Here's how the part is built. I have some questions about the finished solid (model axes, mm). Face numbers are marked on the shaded views. A direction names the side the tool comes from. Coordinates: 2 decimals unless noted, no trailing zeros. Order: outer loops, then holes, each group sorted by start corner. A loop starts at its lowest first (then second) coordinate and runs counter-clockwise, first axis right, second up.
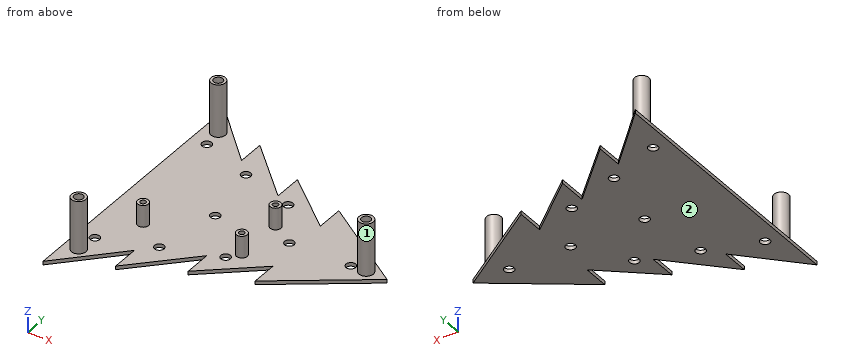
```python
from build123d import *

# Parameters (mm, degrees)
CYLINDER020_R     = 2.55
CYLINDER020_DEPTH = 12
CYLINDER010_R     = 4
CYLINDER010_DEPTH = 31
CYLINDER019_R     = 2.55
CYLINDER019_DEPTH = 12
CYLINDER009_R     = 4
CYLINDER009_DEPTH = 31
CYLINDER018_R     = 2.55
CYLINDER018_DEPTH = 12
CYLINDER011_R     = 4
CYLINDER011_DEPTH = 31
CYLINDER015_R     = 1.55
CYLINDER015_DEPTH = 13
CYLINDER012_R     = 3
CYLINDER012_DEPTH = 13
CYLINDER017_R     = 1.55
CYLINDER017_DEPTH = 13
CYLINDER013_R     = 3
CYLINDER013_DEPTH = 13
CYLINDER008_R     = 2.67
CYLINDER008_DEPTH = 2
CYLINDER007_R     = 2.67
CYLINDER007_DEPTH = 2
CYLINDER006_R     = 2.67
CYLINDER006_DEPTH = 2
CYLINDER005_R     = 2.67
CYLINDER005_DEPTH = 2
CYLINDER004_R     = 2.67
CYLINDER004_DEPTH = 2
CYLINDER003_R     = 2.67
CYLINDER003_DEPTH = 2
CYLINDER002_R     = 2.67
CYLINDER002_DEPTH = 2
CYLINDER001_R     = 2.67
CYLINDER001_DEPTH = 2
CYLINDER_R        = 2.67
CYLINDER_DEPTH    = 3
PAD001_DEPTH      = 2
CYLINDER016_R     = 1.55
CYLINDER016_DEPTH = 13
CYLINDER014_R     = 3
CYLINDER014_DEPTH = 13


with BuildPart() as cylindre002:
    # Cylinder020 → Cylinder020 (new body)
    with BuildSketch(Plane(origin=(-121, 39, 20), x_dir=(1, 0, 0), z_dir=(0, 0, 1))):
        Circle(CYLINDER020_R)
    extrude(amount=CYLINDER020_DEPTH)


with BuildPart() as cut014:
    # Cylinder010 → Cylinder010 (new body)
    with BuildSketch(Plane(origin=(-121, 39, 0), x_dir=(1, 0, 0), z_dir=(0, 0, 1))):
        Circle(CYLINDER010_R)
    extrude(amount=CYLINDER010_DEPTH)

    # Cut014: cut Cylindre002
    add(cylindre002.part, mode=Mode.SUBTRACT)


with BuildPart() as cut014_1:
    # Cut014 placement: moved
    add(cut014.part.moved(Location((-1, 19, 0))))


with BuildPart() as cylindre001:
    # Cylinder019 → Cylinder019 (new body)
    with BuildSketch(Plane(origin=(-2, 0, 20), x_dir=(1, 0, 0), z_dir=(0, 0, 1))):
        Circle(CYLINDER019_R)
    extrude(amount=CYLINDER019_DEPTH)


with BuildPart() as cut013:
    # Cylinder009 → Cylinder009 (new body)
    with BuildSketch(Plane(origin=(-2, 0, 0), x_dir=(1, 0, 0), z_dir=(0, 0, 1))):
        Circle(CYLINDER009_R)
    extrude(amount=CYLINDER009_DEPTH)

    # Cut013: cut Cylindre001
    add(cylindre001.part, mode=Mode.SUBTRACT)


with BuildPart() as cut013_1:
    # Cut013 placement: moved
    add(cut013.part.moved(Location((0.5, 0, 0))))


with BuildPart() as cylindre:
    # Cylinder018 → Cylinder018 (new body)
    with BuildSketch(Plane(origin=(-121, -36, 20), x_dir=(1, 0, 0), z_dir=(0, 0, 1))):
        Circle(CYLINDER018_R)
    extrude(amount=CYLINDER018_DEPTH)


with BuildPart() as cut012:
    # Cylinder011 → Cylinder011 (new body)
    with BuildSketch(Plane(origin=(-121, -36, 0), x_dir=(1, 0, 0), z_dir=(0, 0, 1))):
        Circle(CYLINDER011_R)
    extrude(amount=CYLINDER011_DEPTH)

    # Cut012: cut Cylindre
    add(cylindre.part, mode=Mode.SUBTRACT)


with BuildPart() as cut012_1:
    # Cut012 placement: moved
    add(cut012.part.moved(Location((-1, -22, 0))))


with BuildPart() as arduino_bint:
    # Cylinder015 → Cylinder015 (new body)
    with BuildSketch(Plane(origin=(0, -140, 0), x_dir=(1, 0, 0), z_dir=(0, 0, 1))):
        Circle(CYLINDER015_R)
    extrude(amount=CYLINDER015_DEPTH)


with BuildPart() as arduino_bas:
    # Cylinder012 → Cylinder012 (new body)
    with BuildSketch(Plane(origin=(0, -140, 0), x_dir=(1, 0, 0), z_dir=(0, 0, 1))):
        Circle(CYLINDER012_R)
    extrude(amount=CYLINDER012_DEPTH)

    # Cut: cut Arduino_Bint
    add(arduino_bint.part, mode=Mode.SUBTRACT)


with BuildPart() as arduino_bas_1:
    # Cut placement: moved
    add(arduino_bas.part.moved(Location((-109, 116, 1))))


with BuildPart() as obj1:
    # Cylinder017 → Cylinder017 (new body)
    with BuildSketch(Plane(origin=(0, -140, 0), x_dir=(1, 0, 0), z_dir=(0, 0, 1))):
        Circle(CYLINDER017_R)
    extrude(amount=CYLINDER017_DEPTH)


with BuildPart() as obj2:
    # Cylinder013 → Cylinder013 (new body)
    with BuildSketch(Plane(origin=(0, -140, 0), x_dir=(1, 0, 0), z_dir=(0, 0, 1))):
        Circle(CYLINDER013_R)
    extrude(amount=CYLINDER013_DEPTH)

    # Cut001: cut obj1
    add(obj1.part, mode=Mode.SUBTRACT)


with BuildPart() as obj2_1:
    # Cut001 placement: moved
    add(obj2.part.moved(Location((-57, 148, 1))))


with BuildPart() as obj3:
    # Cylinder008 → Cylinder008 (new body)
    with BuildSketch(Plane(origin=(-85, 0, 0), x_dir=(1, 0, 0), z_dir=(0, 0, 1))):
        Circle(CYLINDER008_R)
    extrude(amount=CYLINDER008_DEPTH)


with BuildPart() as obj4:
    # Cylinder007 → Cylinder007 (new body)
    with BuildSketch(Plane(origin=(-44, 0, 0), x_dir=(1, 0, 0), z_dir=(0, 0, 1))):
        Circle(CYLINDER007_R)
    extrude(amount=CYLINDER007_DEPTH)


with BuildPart() as obj5:
    # Cylinder006 → Cylinder006 (new body)
    with BuildSketch(Plane(origin=(-121, -46, 0), x_dir=(1, 0, 0), z_dir=(0, 0, 1))):
        Circle(CYLINDER006_R)
    extrude(amount=CYLINDER006_DEPTH)


with BuildPart() as obj6:
    # Cylinder005 → Cylinder005 (new body)
    with BuildSketch(Plane(origin=(-92, -36, 0), x_dir=(1, 0, 0), z_dir=(0, 0, 1))):
        Circle(CYLINDER005_R)
    extrude(amount=CYLINDER005_DEPTH)


with BuildPart() as obj7:
    # Cylinder004 → Cylinder004 (new body)
    with BuildSketch(Plane(origin=(-62, -26, 0), x_dir=(1, 0, 0), z_dir=(0, 0, 1))):
        Circle(CYLINDER004_R)
    extrude(amount=CYLINDER004_DEPTH)


with BuildPart() as obj8:
    # Cylinder003 → Cylinder003 (new body)
    with BuildSketch(Plane(origin=(-121, 47, 0), x_dir=(1, 0, 0), z_dir=(0, 0, 1))):
        Circle(CYLINDER003_R)
    extrude(amount=CYLINDER003_DEPTH)


with BuildPart() as obj9:
    # Cylinder002 → Cylinder002 (new body)
    with BuildSketch(Plane(origin=(-92, 36, 0), x_dir=(1, 0, 0), z_dir=(0, 0, 1))):
        Circle(CYLINDER002_R)
    extrude(amount=CYLINDER002_DEPTH)


with BuildPart() as obj10:
    # Cylinder001 → Cylinder001 (new body)
    with BuildSketch(Plane(origin=(-62, 26, 0), x_dir=(1, 0, 0), z_dir=(0, 0, 1))):
        Circle(CYLINDER001_R)
    extrude(amount=CYLINDER001_DEPTH)


with BuildPart() as led_haut:
    # Cylinder → Cylinder (new body)
    with BuildSketch(Plane(origin=(-10, 0, 0), x_dir=(1, 0, 0), z_dir=(0, 0, 1))):
        Circle(CYLINDER_R)
    extrude(amount=CYLINDER_DEPTH)


with BuildPart() as cut011:
    # Sketch → Pad001 (new body)
    with BuildSketch(Plane.XY):
        Polygon((-130.081082, 75.519378), (-130.081082, -75.526209), (-100.046493, -44.621067), (-100.046493, -60.2838), (-69.854797, -29.802717), (-69.854797, -45.272629), (-39.66638, -20.21052), (-39.66638, -34.900669), (10.150305, -0.184029), (-39.87487, 34.909859), (-39.87487, 19.507401), (-70.024222, 45.766594), (-70.024222, 29.628657), (-100.203184, 59.856933), (-100.203184, 44.62989), align=None)
    extrude(amount=PAD001_DEPTH)

    # Cut003: cut Led_haut
    add(led_haut.part, mode=Mode.SUBTRACT)

    # Cut004: cut obj10
    add(obj10.part, mode=Mode.SUBTRACT)

    # Cut005: cut obj9
    add(obj9.part, mode=Mode.SUBTRACT)

    # Cut006: cut obj8
    add(obj8.part, mode=Mode.SUBTRACT)

    # Cut007: cut obj7
    add(obj7.part, mode=Mode.SUBTRACT)

    # Cut008: cut obj6
    add(obj6.part, mode=Mode.SUBTRACT)

    # Cut009: cut obj5
    add(obj5.part, mode=Mode.SUBTRACT)

    # Cut010: cut obj4
    add(obj4.part, mode=Mode.SUBTRACT)

    # Cut011: cut obj3
    add(obj3.part, mode=Mode.SUBTRACT)


with BuildPart() as arduino_dint:
    # Cylinder016 → Cylinder016 (new body)
    with BuildSketch(Plane(origin=(0, -140, 0), x_dir=(1, 0, 0), z_dir=(0, 0, 1))):
        Circle(CYLINDER016_R)
    extrude(amount=CYLINDER016_DEPTH)


with BuildPart() as fusion006:
    # Cylinder014 → Cylinder014 (new body)
    with BuildSketch(Plane(origin=(0, -140, 0), x_dir=(1, 0, 0), z_dir=(0, 0, 1))):
        Circle(CYLINDER014_R)
    extrude(amount=CYLINDER014_DEPTH)

    # Cut002: cut Arduino_Dint
    add(arduino_dint.part, mode=Mode.SUBTRACT)


with BuildPart() as fusion006_1:
    # Cut002 placement: moved
    add(fusion006.part.moved(Location((-57, 120, 1))))

    # Fusion002: union Cut011
    add(cut011.part)

    # Fusion: union obj2
    add(obj2_1.part)

    # Fusion003: union Arduino_bas
    add(arduino_bas_1.part)

    # Fusion004: union Cut012
    add(cut012_1.part)

    # Fusion005: union Cut013
    add(cut013_1.part)

    # Fusion006: union Cut014
    add(cut014_1.part)


solid = fusion006_1.part
```
Q1. For the marked faces 1 and 2, which set-ups out of +Z, -Z, +X, -X, +Y, -Y let a thin tool reach every point of the face, with its end or its side?
Q2. I need wall thicknesses on L1, parallel to Y at x = -57, z = 10; L2, parallel to Y at x = -109, z = 5.75; L3, parallel to Y at x = -121, z = 1. Which ranges of each line are inside material? Lowest first, please.
Q3. If we section it at C-C on y = 31.5: Write out the boundary of the cut face in (x, z).
Q4. If we section it at B-B on y = -58: Write out the boundary of the cut face in (x, z).
Q5. If we section it at A-A on z = 6: Give the number of separate pieces and of enclosed holes in the cut face, then the cut area to 3 significant figures.
Q6. Will these pins go through, and if not, where does the flat tip stop? pin 1 (1.5 mm diameter, centred on x = -2.5, y = -0.5, fed in from +Z); pin 2 (1.5 mm diameter, centred on x = -109.5, y = -24.5, fed in from +Z); pin 3 (12 mm diameter, centred on x = -35, z = 13.5, fed in from -Y); pin 4 (2.5 mm diameter, centred on x = -57.5, y = -20, fed in from +Z).
Q7. If we section it at D-D on x = -10: Write out the boundary of the cut face in (y, z).
Reply:
1. face 1: +Z
1. face 2: -Z, +X, -X, +Y, -Y
2. L1: y = -23 to -21.55, -18.45 to -17, 5 to 6.45, 9.55 to 11
2. L2: y = -27 to -25.55, -22.45 to -21
2. L3: y = -66.18 to -48.67, -43.33 to 44.33, 49.67 to 66.13
3. outline: (-130.08, 0) - (-71.89, 0) - (-71.89, 2) - (-130.08, 2) - close; (-70.02, 0) - (-53.64, 0) - (-53.64, 2) - (-70.02, 2) - close; (-39.87, 0) - (-35.01, 0) - (-35.01, 2) - (-39.87, 2) - close
4. outline: (-130.08, 0) - (-113.05, 0) - (-113.05, 2) - (-118, 2) - (-118, 31) - (-119.45, 31) - (-119.45, 20) - (-124.55, 20) - (-124.55, 31) - (-126, 31) - (-126, 2) - (-130.08, 2) - close; (-100.05, 0) - (-97.78, 0) - (-97.78, 2) - (-100.05, 2) - close
5. separate pieces: 6
5. enclosed holes: 3
5. area: 213 mm2
6. pin 1: stops at z = 20
6. pin 2: stops at z = 2
6. pin 3: passes through
6. pin 4: stops at z = 14
7. outline: (-14.23, 0) - (-2.67, 0) - (-2.67, 2) - (-14.23, 2) - close; (2.67, 0) - (13.95, 0) - (13.95, 2) - (2.67, 2) - close
